from build123d import *

# Parameters (mm, degrees)
SKETCH1_R               = 10.25
SKETCH1_R_2             = 8.5
BOSS_EXTRUDE1_DEPTH     = 5
CUT_EXTRUDE1_START      = -10.2500001
CUT_EXTRUDE1_OUTLINE_W  = 20.5
CUT_EXTRUDE1_OUTLINE_H  = 5
CUT_EXTRUDE1_DEPTH      = 17.878072963
CUT_EXTRUDE1_START_2    = 7.628072863
CUT_EXTRUDE1_2_DEPTH    = 2.545422212
CUT_EXTRUDE7_REACH      = 26.005
CUT_EXTRUDE7_END_RADIUS = 9.1
CUT_EXTRUDE7_START      = 12
SKETCH3_W               = 3
SKETCH3_H               = 1.8
CUT_EXTRUDE8_DEPTH      = 8.8


# Read off the part's stored shape, not the designer's step: Cut-Extrude1
with BuildPart() as part:
    # Sketch1 → Boss-Extrude1 (new body)
    with BuildSketch(Plane(origin=(0, 0, 0), x_dir=(1, 0, 0), z_dir=(0, 1, 0))):
        with Locations(Location((0, 0, 0), (0, 0, 270))):
            Circle(SKETCH1_R)
        with Locations(Location((0, 0, 0), (0, 0, 270))):
            Circle(SKETCH1_R_2, mode=Mode.SUBTRACT)
    extrude(amount=BOSS_EXTRUDE1_DEPTH)

    # Cut-Extrude1 outline → Cut-Extrude1 (cut)
    with BuildSketch(Plane.XY.offset(CUT_EXTRUDE1_START)):
        with Locations((0, 2.5)):
            Rectangle(CUT_EXTRUDE1_OUTLINE_W, CUT_EXTRUDE1_OUTLINE_H)
    extrude(amount=CUT_EXTRUDE1_DEPTH, mode=Mode.SUBTRACT)

    # Cut-Extrude1 2 outline → Cut-Extrude1 2 (cut)
    with BuildSketch(Plane.XY.offset(CUT_EXTRUDE1_START_2)):
        with BuildLine():
            ThreePointArc((-3.75, 2.5), (-3.017766953, 4.267766953), (-1.25, 5))
            Line((-1.25, 5), (-10.25, 5))
            Line((-10.25, 5), (-10.25, 0))
            Line((-10.25, 0), (-3.75, 0))
            Line((-3.75, 0), (-3.75, 2.5))
        make_face()
        with BuildLine():
            Line((10.25, 5), (1.25, 5))
            ThreePointArc((1.25, 5), (3.017766953, 4.267766953), (3.75, 2.5))
            Line((3.75, 2.5), (3.75, 0))
            Line((3.75, 0), (10.25, 0))
            Line((10.25, 0), (10.25, 5))
        make_face()
    extrude(amount=CUT_EXTRUDE1_2_DEPTH, mode=Mode.SUBTRACT)

    # Cut-Extrude7: up to this cylinder (the profile starts outside it)
    cut_extrude7_end = Plane(origin=(0, 2.7341405, 0), z_dir=(0, -1, 0)) * Cylinder(CUT_EXTRUDE7_END_RADIUS, 75.561441, mode=Mode.PRIVATE)
    # Sketch2<4> → Cut-Extrude7 (cut, up to the surface)
    with BuildSketch(Plane.XY.offset(CUT_EXTRUDE7_START), mode=Mode.PRIVATE) as cut_extrude7_sk1:
        with BuildLine():
            Line((1.25, 5), (-1.25, 5))
            ThreePointArc((-1.25, 5), (-3.017766953, 4.267766953), (-3.75, 2.5))
            ThreePointArc((-3.75, 2.5), (-3.017766953, 0.732233047), (-1.25, 0))
            Line((-1.25, 0), (1.25, 0))
            ThreePointArc((1.25, 0), (3.017766953, 0.732233047), (3.75, 2.5))
            ThreePointArc((3.75, 2.5), (3.017766953, 4.267766953), (1.25, 5))
        make_face()
        with BuildLine():
            ThreePointArc((-2.75, 2.5), (-2.310660172, 3.560660172), (-1.25, 4))
            Line((-1.25, 4), (1.25, 4))
            ThreePointArc((1.25, 4), (2.310660172, 3.560660172), (2.75, 2.5))
            Line((2.75, 2.5), (2.75, 1))
            Line((2.75, 1), (1.25, 1))
            Line((1.25, 1), (-1.25, 1))
            Line((-1.25, 1), (-2.75, 1))
            Line((-2.75, 1), (-2.75, 2.5))
        make_face(mode=Mode.SUBTRACT)
    cut_extrude7_tool1 = extrude(cut_extrude7_sk1.sketch, amount=-CUT_EXTRUDE7_REACH, mode=Mode.PRIVATE) - cut_extrude7_end
    add(cut_extrude7_tool1.solids().sort_by_distance((0, 4.909861, 12))[0], mode=Mode.SUBTRACT)
    # Sketch2<4> → Cut-Extrude7 (cut, up to the surface)
    with BuildSketch(Plane.XY.offset(CUT_EXTRUDE7_START), mode=Mode.PRIVATE) as cut_extrude7_sk2:
        with BuildLine():
            ThreePointArc((-1.25, 0), (-3.017766953, 0.732233047), (-3.75, 2.5))
            Line((-3.75, 2.5), (-3.75, 0))
            Line((-3.75, 0), (-1.25, 0))
        make_face()
    cut_extrude7_tool2 = extrude(cut_extrude7_sk2.sketch, amount=-CUT_EXTRUDE7_REACH, mode=Mode.PRIVATE) - cut_extrude7_end
    add(cut_extrude7_tool2.solids().sort_by_distance((-3.19158, 0.55842, 12))[0], mode=Mode.SUBTRACT)
    # Sketch2<4> → Cut-Extrude7 (cut, up to the surface)
    with BuildSketch(Plane.XY.offset(CUT_EXTRUDE7_START), mode=Mode.PRIVATE) as cut_extrude7_sk3:
        with BuildLine():
            Line((3.75, 0), (3.75, 2.5))
            ThreePointArc((3.75, 2.5), (3.017766953, 0.732233047), (1.25, 0))
            Line((1.25, 0), (3.75, 0))
        make_face()
    cut_extrude7_tool3 = extrude(cut_extrude7_sk3.sketch, amount=-CUT_EXTRUDE7_REACH, mode=Mode.PRIVATE) - cut_extrude7_end
    add(cut_extrude7_tool3.solids().sort_by_distance((3.19158, 0.55842, 12))[0], mode=Mode.SUBTRACT)

    # Sketch3 → Cut-Extrude8 (cut)
    with BuildSketch(Plane.XY):
        with Locations((0, 2.4)):
            Rectangle(SKETCH3_W, SKETCH3_H)
    extrude(amount=CUT_EXTRUDE8_DEPTH, mode=Mode.SUBTRACT)


solid = part.part
Source: CAD feature listing. Evaluate the final solid. Frame: model axes, mm. A direction names the side the tool comes from. Round coordinates to 2 decimals unless told otherwise and drop trailing zeros. Loops run counter-clockwise (first coordinate to the right, second up) from the corner with the lowest first, then second, coordinate; pieces in that order, holes last. Notation, with made-up numbers: (-27, -38) - (22, -38) arc R32 cw to (22, -10) - close; hole circle Ø6 at (76.25, -25.5). An arc over 180 degrees is marked (long way). Write item = value, one per line. Start each with the question number.
Item 1: Section query D-D on y = 2.8. Output: boundary loops of the cut face in (x, z), plus the area to 3 significant figures.
Item 2: Mould query, pull axis Y, two halves, no side actions, for faces 1 (the face through (2.75, 2, 9)), 2 (the face through (2.998, 4.287, 8.311)), 3 (the face through (0, 2, 8.8)). Classes: released by +Y, released by -Y, zero draft, split by the parting line, or undercut.
Item 3: Section query A-A on z = 9.65. Output: boundary loops of the cut face in (x, y), plus the area to 3 significant figures.
Item 4: Section query B-B on y = 2.25. Output: boundary loops of the cut face in (x, z).
Item 5: Material intervals for line 1 (Y direction, x = 1.25, z = 8.6); line 2 (Z direction, x = 1.25, y = 2.7); line 3 (Y direction, x = -0.75, z = 9.55), sorted ascending.
Item 6: Reachability of faces 4 (the face through (-2.75, 2, 9)), 5 (the face through (-2.32, 3.55, 9.43)), 6 (the face through (2.3, 3.57, 9.43)), 7 (the face through (-0.04, 2.48, 10.25)) from +Z, -Z, +X, -X, +Y, -Y: full face, straight path, thin tool, end or side. Return the list, or none.
Item 7: First-contact query: pin 1 Ø1.5 at (x, z) = (0.5, 8.5) entering from -Y; pin 2 Ø1.4 at (x, y) = (0, 2) entering from -Z. Flat tips, straight axial feed; report the tip coordinate or a pass-through.
Item 8: Section query C-C on x = 2. Output: boundary loops of the cut face in (y, z).
Results list:
q1.outline = (-3.73, 7.64) arc R8.5 cw to (-1.5, 8.37) - (-1.5, 8.8) - (1.5, 8.8) - (1.5, 8.37) arc R8.5 cw to (3.73, 7.64) - (3.73, 8.3) arc R9.1 ccw to (2.72, 8.68) - (2.72, 9.88) arc R10.25 ccw to (-2.72, 9.88) - (-2.72, 8.68) arc R9.1 ccw to (-3.73, 8.3) - close
q1.area = 9.93 mm²
q2.face_1 = zero draft
q2.face_2 = released by +Y
q2.face_3 = undercut
q3.outline = (-2.75, 1) - (2.75, 1) - (2.75, 2.5) arc R1.5 ccw to (1.25, 4) - (-1.25, 4) arc R1.5 ccw to (-2.75, 2.5) - close
q3.area = 15.5 mm²
q4.outline = (-3.75, 7.63) arc R8.5 cw to (-1.5, 8.37) - (-1.5, 8.8) - (1.5, 8.8) - (1.5, 8.37) arc R8.5 cw to (3.75, 7.63) - (3.75, 8.29) arc R9.1 ccw to (2.75, 8.67) - (2.75, 9.87) arc R10.25 ccw to (-2.75, 9.87) - (-2.75, 8.67) arc R9.1 ccw to (-3.75, 8.29) - close
q5.line_1 = 0 to 1.5, 3.3 to 5
q5.line_2 = 8.8 to 10.17
q5.line_3 = 1 to 4
q6.face_4 = +Z, -X, +Y, -Y
q6.face_5 = +Z, -X, +Y
q6.face_6 = +Z, +X, +Y
q6.face_7 = +Z, +Y, -Y
q7.pin_1 = 0
q7.pin_2 = 8.49
q8.outline = (0, 8.26) - (4.88, 8.26) - (4.88, 8.88) - (3.8, 8.88) - (3.8, 10.05) - (1, 10.05) - (1, 8.88) - (0, 8.88) - close
